```python
from build123d import *

# Parameters (mm, degrees)
CUT_EXTRUDE_1_DEPTH = 2


with BuildPart() as part:
    # Sketch 1 → Revolve 1 (revolve)
    with BuildSketch(Plane.XY, mode=Mode.PRIVATE) as revolve_1_sk:
        Polygon((-4, 0), (-4, 3.5), (0, 3.5), (0, 2), (19.5, 2), (20, 1.5), (20, 0), align=None)
    revolve(revolve_1_sk.sketch.rotate(Axis((20, 0, 0), (-1, 0, 0)), 180), axis=Axis((20, 0, 0), (-1, 0, 0)))

    # Sketch 2 → Cut-Revolve 1 (revolve, cut)
    with BuildSketch(Plane.XY, mode=Mode.PRIVATE) as cut_revolve_1_sk:
        Polygon((-4, 0), (-4, 1.5), (-2, 1.5), (-1.598076211, 0), align=None)
    revolve(cut_revolve_1_sk.sketch.rotate(Axis((-1.598076211, 0, 0), (-1, 0, 0)), 270), axis=Axis((-1.598076211, 0, 0), (-1, 0, 0)), mode=Mode.SUBTRACT)

    # Sketch 3 → Cut-Extrude 1 (cut)
    with BuildSketch(Plane(origin=(-4, 0, 0), x_dir=(0, 0, -1), z_dir=(1, 0, 0))):
        Polygon((-1.5, 0.866025404), (-1.5, -0.866025404), (0, -1.732050808), (1.5, -0.866025404), (1.5, 0.866025404), (0, 1.732050808), align=None)
    extrude(amount=CUT_EXTRUDE_1_DEPTH, mode=Mode.SUBTRACT)


solid = part.part
```
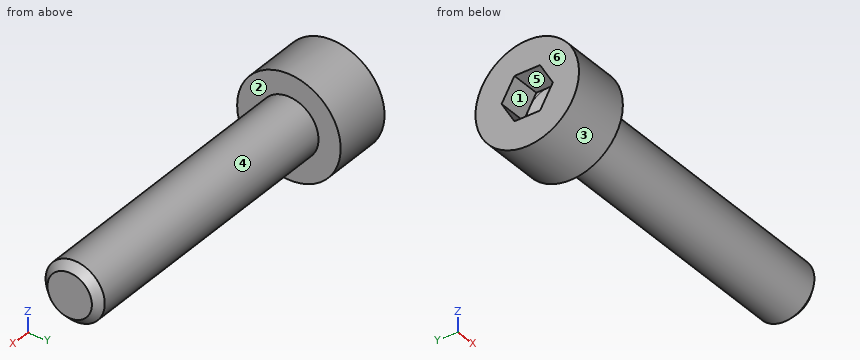
Can you work these out from the model? Positions are in its coordinate system, mm. Face numbers are marked on the shaded views. A direction names the side the tool comes from. Coordinates: 2 decimals unless noted, no trailing zeros. Loops run counter-clockwise (first coordinate to the right, second up) from the corner with the lowest first, then second, coordinate; pieces in that order, holes last. Notation, with made-up numbers: (16, -4) -> (34, -4) arc R17 ccw to (34, 22) -> close; hole circle Ø4 at (60.25, 54.25). An arc over 180 degrees is marked (long way). Answer as a JSON object with one key per item and string values.
1) Thinking about a two-plate mould opening in Y: for the marked faces 1, 2 and 3, which applies, pulls with the +Y half, pulls with the -Y half, needs draft (parallel to the pull), parting line crosses it, or undercut?
Results:
{"face 1": "undercut", "face 2": "needs draft", "face 3": "parting line crosses it"}
2) Imagine slicing it at B-B (y = 2.75). Please give me the cut outline in (x, z).
Results:
{"outline": "(-4, -2.17) -> (0, -2.17) -> (0, 2.17) -> (-4, 2.17) -> close"}
3) Imagine slicing it at A-A (x = 3.75). Please give me the cut outline in (y, z).
Results:
{"outline": "circle Ø4 at (0, 0)"}
4) If I drill on line 1 (X direction, y = -2, z = 0.5); line 2 (Y direction, x = 15, z = -1); line 3 (Y direction, x = 9.75, z = -0.5), over which ranges is the centre line in solid material (lowest first)?
Results:
{"line 1": "x = -4 to 0", "line 2": "y = -1.73 to 1.73", "line 3": "y = -1.94 to 1.94"}
5) For the marked faces 4, 5 and 6, which set-ups out of +Z, -Z, +X, -X, +Y, -Y let a thin tool reach every point of the face, with its end or its side?
Results:
{"face 4": "+X", "face 5": "-X", "face 6": "+Z, -Z, -X, +Y, -Y"}
6) For P1, Ø2, axis at y = 2.5, z = 1.5, coming from the +X side; P2, Ø0.8, axis at y = 0.5, z = -1, coming from the -X side; P3, Ø1, axis at x = 16.5, z = -1, coming from the -Y side, each with a flat end and sliding along its axis, tell me the tip position at first contact or that it passes through.
Results:
{"P1": "stops at x = 19.58", "P2": "stops at x = -2", "P3": "stops at y = -1.94"}
